Verification items for this drawing (mm, ordinates from the low corner). Coordinates: 2 decimals unless noted, no trailing zeros. Order: outer loops, then holes, each group sorted by start corner. A loop starts at its lowest first (then second) coordinate and runs counter-clockwise, first axis right, second up. Notation, with made-up numbers: (-11.75, -37) - (5.25, -37) arc R25 cw to (5.25, -20) - close; hole circle Ø11 at (54.5, -36). An arc over 180 degrees is marked (long way). One line per question, with ' | ' between items. Start each with the question number.
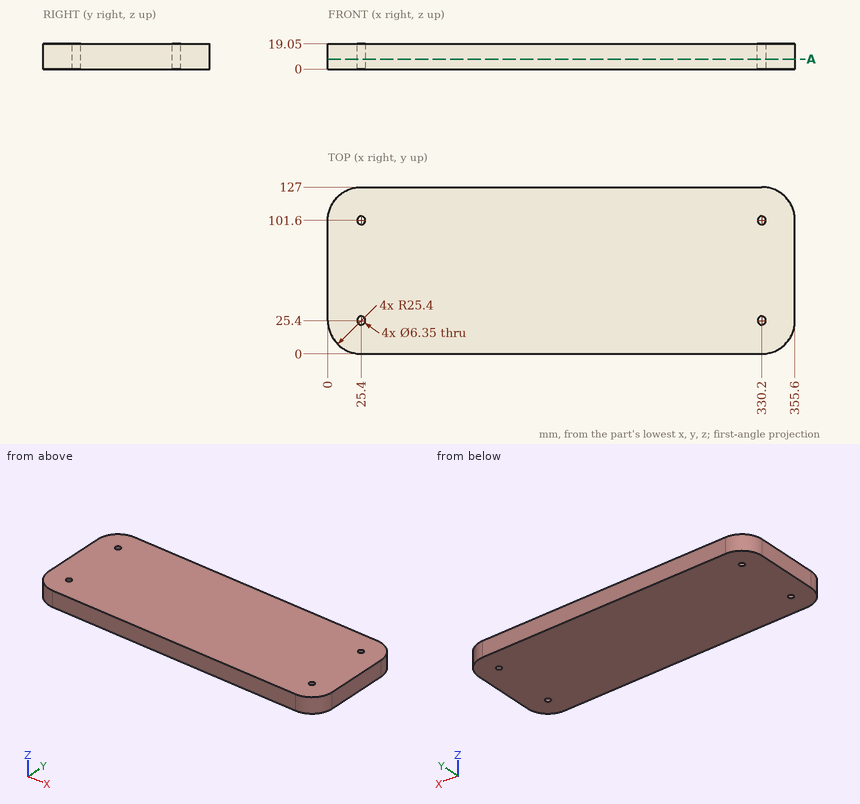
Item 1: Section check A-A (z = 7.5). Record the cut outline in (x, y) (3 decimals), then the cut area to 3 significant figures.
Item 2: Gauge pin test, flat ends, axial feed: pin 1 (4 mm diameter, centred on y = 73, z = 17, fed in from -X); pin 2 (4 mm diameter, centred on y = 110, z = 9.5, fed in from -X); pin 3 (5.5 mm diameter, centred on x = 25.4, y = 25.4, fed in from +Z); pin 4 (8 mm diameter, centred on y = 21, z = 14, fed in from +X). Record the tip position at first contact, or that the pin passes through.
Item 3: Thickness scan on probe 1 along X at (y, z) = (26, 10.25); probe 2 along X at (y, z) = (102.5, 16.5); probe 3 along X at (y, z) = (19, 11.5). Record the ranges inside material, lowest first. Write a range as from..to.
Completed:
1) outline: (0, 25.4) arc R25.4 ccw to (25.4, 0) - (330.2, 0) arc R25.4 ccw to (355.6, 25.4) - (355.6, 101.6) arc R25.4 ccw to (330.2, 127) - (25.4, 127) arc R25.4 ccw to (0, 101.6) - close; hole circle Ø6.35 at (25.4, 25.4); hole circle Ø6.35 at (25.4, 101.6); hole circle Ø6.35 at (330.2, 25.4); hole circle Ø6.35 at (330.2, 101.6) | area: 44,500 mm^2
2) pin 1: stops at x = 0 | pin 2: stops at x = 0.82 | pin 3: passes through | pin 4: stops at x = 355.6
3) probe 1: x = 0..22.28, 28.52..327.08, 333.32..355.6 | probe 2: x = 0.02..22.36, 28.44..327.16, 333.24..355.58 | probe 3: x = 0.82..354.78
